from build123d import *

# Parameters (mm, degrees)
EXTRUDE_1_DEPTH     = 25
SKETCH_2_R          = 3.2
CUT_EXTRUDE_1_DEPTH = 35
SKETCH_3_R          = 3.2
CUT_EXTRUDE_2_DEPTH = 35
SKETCH_5_W          = 22.25
SKETCH_5_H          = 22.25
CUT_EXTRUDE_4_DEPTH = 25
EXTRUDE_2_DEPTH     = 20
SKETCH_7_R          = 2.7
CUT_EXTRUDE_5_DEPTH = 5
SKETCH_8_R          = 2.7
CUT_EXTRUDE_6_DEPTH = 5
FILLET_1_R          = 2


with BuildPart() as part:
    # 스케치1 → 보스-돌출1 (new body)
    with BuildSketch(Plane(origin=(0, 0, 0), x_dir=(1, 0, 0), z_dir=(0, 1, 0))):
        Polygon((-17.5, 68.5), (-11.25, 68.5), (-11.25, 38.5), (11.25, 38.5), (11.25, 68.5), (17.5, 68.5), (17.5, -17.5), (-68.5, -17.5), (-68.5, -11.25), (-38.5, -11.25), (-38.5, 11.25), (-68.5, 11.25), (-68.5, 17.5), (-17.5, 17.5), align=None)
    extrude(amount=EXTRUDE_1_DEPTH)

    # 스케치2 → 컷-돌출1 (cut)
    with BuildSketch(Plane(origin=(17.5, 0, 0), x_dir=(0, 0, -1), z_dir=(1, 0, 0))):
        with Locations((61, 12.5)):
            Circle(SKETCH_2_R)
        with Locations((46, 12.5)):
            Circle(SKETCH_2_R)
    extrude(amount=-CUT_EXTRUDE_1_DEPTH, mode=Mode.SUBTRACT)

    # 스케치3 → 컷-돌출2 (cut)
    with BuildSketch(Plane.XY.offset(17.5)):
        with Locations((-61, 12.5)):
            Circle(SKETCH_3_R)
        with Locations((-46, 12.5)):
            Circle(SKETCH_3_R)
    extrude(amount=-CUT_EXTRUDE_2_DEPTH, mode=Mode.SUBTRACT)

    # 스케치5 → 컷-돌출4 (cut)
    with BuildSketch(Plane(origin=(0, 25, 0), x_dir=(1, 0, 0), z_dir=(0, 1, 0))):
        with Locations((6.375, -6.375)):
            Rectangle(SKETCH_5_W, SKETCH_5_H)
    extrude(amount=-CUT_EXTRUDE_4_DEPTH, mode=Mode.SUBTRACT)

    # 스케치6 → 보스-돌출2 (add)
    with BuildSketch(Plane.XZ):
        Polygon((-9.75, 17.5), (-4.75, 17.5), (-4.75, -4.75), (17.5, -4.75), (17.5, -9.75), (-9.75, -9.75), align=None)
    extrude(amount=EXTRUDE_2_DEPTH)

    # 스케치7 → 컷-돌출5 (cut)
    with BuildSketch(Plane(origin=(-4.75, 0, 0), x_dir=(0, 0, -1), z_dir=(1, 0, 0))):
        with Locations((-5.25, -10)):
            Circle(SKETCH_7_R)
    extrude(amount=-CUT_EXTRUDE_5_DEPTH, mode=Mode.SUBTRACT)

    # 스케치8 → 컷-돌출6 (cut)
    with BuildSketch(Plane.XY.offset(-4.75)):
        with Locations((5.25, -10)):
            Circle(SKETCH_8_R)
    extrude(amount=-CUT_EXTRUDE_6_DEPTH, mode=Mode.SUBTRACT)

    # 필렛1
    fillet_1_edges = [part.edges().sort_by_distance(p)[0] for p in [
        (-17.5, 12.5, -68.5),
        (17.5, 12.5, -68.5),
        (-68.5, 12.5, 17.5),
        (-68.5, 12.5, -17.5),
        (-17.5, 12.5, -17.5),
        (-4.75, 2.5, 17.5),
        (17.5, 2.5, -4.75),
        (-9.75, 0, 3.875),
        (3.875, 0, -9.75),
        (-9.75, -10, -9.75),
    ]]
    fillet(fillet_1_edges, radius=FILLET_1_R)


solid = part.part
Source: CAD feature listing. Evaluate the final solid. Frame: model axes, mm. A direction names the side the tool comes from. Give positions to 0.01 mm unless a question says otherwise; leave off trailing zeros. Write each loop counter-clockwise with the first axis right and the second up, starting at its lowest first coordinate (ties: lowest second). Pieces come first, ordered by that corner, then holes. Notation, with made-up numbers: M 33.5,11 L 91.5,11 A26 ccw 91.5,41 Z; hole C 46.25,48 d9. An arc over 180 degrees is marked long. Answer as a JSON object with one key per item and string values.
Q1. Cut plane D-D, the plane z = -51. Return the cut outline in (x, y), then the cut area to 4 significant figures.
Geometry check:
{"outline": "M -17.5,0 L -11.25,0 L -11.25,25 L -17.5,25 Z; M 11.25,0 L 17.5,0 L 17.5,25 L 11.25,25 Z", "area": "312.5 mm^2"}
Q2. Cut plane B-B, the plane x = -61. Return the cut outline in (y, z).
Geometry check:
{"outline": "M 0,-17.5 L 9.3,-17.5 L 9.3,-11.25 L 0,-11.25 Z; M 0,11.25 L 9.3,11.25 L 9.3,17.5 L 0,17.5 Z; M 15.7,-17.5 L 25,-17.5 L 25,-11.25 L 15.7,-11.25 Z; M 15.7,11.25 L 25,11.25 L 25,17.5 L 15.7,17.5 Z"}
Q3. Ray query, line 1 along X through (y, z) = (21, -51); line 2 along Y through (x, z) = (-7, 5). Return the intervals inside material, ascending.
Geometry check:
{"line 1": "x = -17.5 to -11.25, 11.25 to 17.5", "line 2": "y = -20 to -12.69, -7.31 to 25"}
Q4. Cut plane C-C, the plane y = -10. Return the cut outline in (x, z), then the cut area to 3 significant figures.
Geometry check:
{"outline": "M -9.75,-7.75 A2 ccw -7.75,-9.75 L 2.55,-9.75 L 2.55,-4.75 L -4.75,-4.75 L -4.75,2.55 L -9.75,2.55 Z; M -9.75,7.95 L -4.75,7.95 L -4.75,15.5 A2 ccw -6.75,17.5 L -9.75,17.5 Z; M 7.95,-9.75 L 17.5,-9.75 L 17.5,-6.75 A2 ccw 15.5,-4.75 L 7.95,-4.75 Z", "area": "191 mm^2"}
Q5. Mould query, pull axis Y, two halves, no side actions, for faces 1 (the face through (-11.25, 12, -54)), 2 (the face through (-15, 0, -17)), 3 (the face through (14.419, 9.661, -47.477)). Classes: +Y half, -Y half, draft (parallel to the pull), parting line (faces both ways), or undercut.
Geometry check:
{"face 1": "draft", "face 2": "-Y half", "face 3": "undercut"}
Q6. Access query for faces 4 (the face through (-17.5, 10, -43)), 5 (the face through (-44.523, 9.661, -14.331)), 6 (the face through (-54, 12, 11.25)), 7 (the face through (14.419, 10.553, -58.461)), 8 (the face through (5, 3, -4.75)). Directions: +Z, -Z, +X, -X, +Y, -Y. A direction counts if a zero-diameter tool reaches every point of the face in a straight line with its end or side. Return the directions, or none.
Geometry check:
{"face 4": "-Z, -X, +Y, -Y", "face 5": "+Z, -Z", "face 6": "-X, +Y, -Y", "face 7": "+X, -X", "face 8": "+Z, +X, +Y, -Y"}
Q7. Contact query for flat-ended pins moving along their axis: P1, Ø6, axis at y = -10, z = 5.25, coming from the +X side; P2, Ø20, axis at x = 6, y = -12, coming from the -Z side; P3, Ø14.5, axis at y = -9.5, z = 11, coming from the -X side. Output: stop coordinate, or through.
Geometry check:
{"P1": "stops at x = -4.75", "P2": "stops at z = -9.75", "P3": "stops at x = -9.75"}
Q8. Cut plane A-A, the plane z = -61. Return the cut outline in (x, y).
Geometry check:
{"outline": "M -17.5,0 L -11.25,0 L -11.25,9.3 L -17.5,9.3 Z; M -17.5,15.7 L -11.25,15.7 L -11.25,25 L -17.5,25 Z; M 11.25,0 L 17.5,0 L 17.5,9.3 L 11.25,9.3 Z; M 11.25,15.7 L 17.5,15.7 L 17.5,25 L 11.25,25 Z"}
